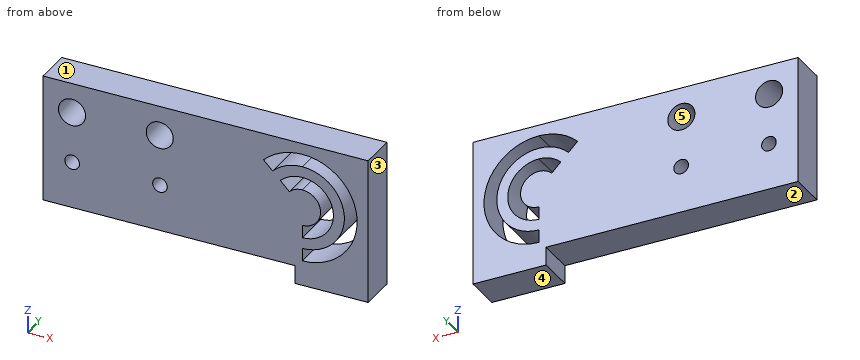
```python
from build123d import *

# Parameters (mm, degrees)
F0_R     = 1
F0_R_2   = 1.85
F1_DEPTH = 5


with BuildPart() as f1:
    # F0 (on Front) → F1 (new body)
    with BuildSketch(Plane.XZ):
        Polygon((10, 0), (10, 19.95), (1, 19.95), (-34.47, 19.95), (-34.47, 2.5), (-30.48, 2.5), (0.02, 2.5), (0, 0), align=None)
        with Locations((-30.48, 8.88)):
            Circle(F0_R, mode=Mode.SUBTRACT)
        with Locations((-18.47, 8.88)):
            Circle(F0_R, mode=Mode.SUBTRACT)
        with Locations((-30.5, 15.89)):
            Circle(F0_R_2, mode=Mode.SUBTRACT)
        with Locations((-18.5, 15.89)):
            Circle(F0_R_2, mode=Mode.SUBTRACT)
        with BuildLine():
            ThreePointArc((-2.005204, 13.955204), (-0.626405, 14.876488), (1, 15.2))
            ThreePointArc((1, 15.2), (5.25, 10.95), (1, 6.7))
            Line((1, 6.7), (1, 8.45))
            ThreePointArc((1, 8.45), (3.5, 10.95), (1, 13.45))
            ThreePointArc((1, 13.45), (0.043291, 13.259699), (-0.767767, 12.717767))
            Line((-0.767767, 12.717767), (-2.005204, 13.955204))
        make_face(mode=Mode.SUBTRACT)
        with BuildLine():
            ThreePointArc((-4.303301, 16.253301), (-1.870126, 17.879096), (1, 18.45))
            ThreePointArc((1, 18.45), (8.5, 10.95), (1, 3.45))
            Line((1, 3.45), (1, 5.2))
            ThreePointArc((1, 5.2), (6.75, 10.95), (1, 16.7))
            ThreePointArc((1, 16.7), (-1.20043, 16.262307), (-3.065864, 15.015864))
            Line((-3.065864, 15.015864), (-4.303301, 16.253301))
        make_face(mode=Mode.SUBTRACT)
    extrude(amount=-F1_DEPTH)


solid = f1.part
```
Design review of the part built by this model. Coordinates are the model's own, in mm. Face numbers are marked on the shaded views. A direction names the side the tool comes from. Round coordinates to 2 decimals unless told otherwise and drop trailing zeros. Write each loop counter-clockwise with the first axis right and the second up, starting at its lowest first coordinate (ties: lowest second). Pieces come first, ordered by that corner, then holes. Notation, with made-up numbers: (66, 16) -> (102, 16) arc R9 ccw to (102, 30) -> close; hole circle Ø7 at (-17, -5). An arc over 180 degrees is marked (long way). Write item = value, one per line. Start each with the question number.
1) Tool access review of the marked faces 1 and 2: name each direction out of +Z, -Z, +X, -X, +Y, -Y from which nothing blocks a thin tool from reaching the whole face with its end or side.
2) Take a section at D-D, the plane y = 1.75. State the section outline as (x, z) points.
3) Wall thickness on probe 1 along Z at (x, y) = (-30.48, 2.05); probe 2 along X at (y, z) = (1.9, 14); probe 3 along Z at (x, y) = (4, 4.6): over which ranges is each line inside the solid? List them lowest first. Write a range as from..to.
4) Take a section at B-B, the plane x = -30.5. State the section outline as (y, z) points, plus the area to 3 significant figures.
5) Take a section at C-C, the plane z = 8.88. State the section outline as (x, y) points, plus the area to 3 significant figures.
6) Mouldability with a two-part tool opening along Z and no side actions: class the marked faces 3, 4 and 5 as +Z half, -Z half, draft (parallel to the pull), parting line (faces both ways), or undercut.
7) Take a section at A-A, the plane z = 10.95. State the section outline as (x, y) points.
8) Clearance check with flat-ended pins moving along their axes: pin 1 (1 mm diameter, centred on x = -17.5, y = 3.5, fed in from -Z); pin 2 (3.5 mm diameter, centred on x = -18.5, z = 15.89, fed in from +Y). State where each tip first meets the part, or that it passes through.
Results list:
q1.face_1 = +Z, +X, -X, +Y, -Y
q1.face_2 = -Z, -X, +Y, -Y
q2.outline = (-34.47, 2.5) -> (0.02, 2.5) -> (0, 0) -> (10, 0) -> (10, 19.95) -> (-34.47, 19.95) -> close; hole circle Ø3.7 at (-30.5, 15.89); hole circle Ø2 at (-30.48, 8.88); hole circle Ø3.7 at (-18.5, 15.89); hole circle Ø2 at (-18.47, 8.88); hole (-4.3, 16.25) -> (-3.07, 15.02) arc R5.75 cw to (1, 16.7) arc R5.75 cw to (1, 5.2) -> (1, 3.45) arc R7.5 ccw to (1, 18.45) arc R7.5 ccw to start; hole (-2.01, 13.96) -> (-0.77, 12.72) arc R2.5 cw to (1, 13.45) arc R2.5 cw to (1, 8.45) -> (1, 6.7) arc R4.25 ccw (long way) to start
q3.probe_1 = 2.5..7.88, 9.88..14.04, 17.74..19.95
q3.probe_2 = -34.47..-1.96, 3.96..5.87, 7.85..10
q3.probe_3 = 0..4.08, 6.04..7.94, 13.96..15.86, 17.82..19.95
q4.outline = (0, 2.5) -> (5, 2.5) -> (5, 7.88) -> (0, 7.88) -> close; (0, 9.88) -> (5, 9.88) -> (5, 14.04) -> (0, 14.04) -> close; (0, 17.74) -> (5, 17.74) -> (5, 19.95) -> (0, 19.95) -> close
q4.area = 58.8 mm²
q5.outline = (-34.47, 0) -> (-31.48, 0) -> (-31.48, 5) -> (-34.47, 5) -> close; (-29.48, 0) -> (-19.47, 0) -> (-19.47, 5) -> (-29.48, 5) -> close; (-17.47, 0) -> (2.4, 0) -> (2.4, 5) -> (-17.47, 5) -> close; (4.71, 0) -> (6.36, 0) -> (6.36, 5) -> (4.71, 5) -> close; (8.21, 0) -> (10, 0) -> (10, 5) -> (8.21, 5) -> close
q5.area = 182 mm²
q6.face_3 = draft
q6.face_4 = -Z half
q6.face_5 = undercut
q7.outline = (-34.47, 0) -> (3.5, 0) -> (3.5, 5) -> (-34.47, 5) -> close; (5.25, 0) -> (6.75, 0) -> (6.75, 5) -> (5.25, 5) -> close; (8.5, 0) -> (10, 0) -> (10, 5) -> (8.5, 5) -> close
q8.pin_1 = 2.5
q8.pin_2 = through
